Source: CAD feature listing. Evaluate the final solid. Frame: model axes, mm. Coordinates: 2 decimals unless noted, no trailing zeros. Order: outer loops, then holes, each group sorted by start corner. A loop starts at its lowest first (then second) coordinate and runs counter-clockwise, first axis right, second up. Notation, with made-up numbers: (12, 86.25) -> (45, 86.25) arc R19 ccw to (45, 104.25) -> close; hole circle Ø11 at (44.25, 40.25). An arc over 180 degrees is marked (long way). Write each question's results on one line, items separated by ' | '. Start each with the question number.
from build123d import *


with BuildPart() as part:
    # Sketch1 → Revolve1 (revolve)
    with BuildSketch(Plane.XY, mode=Mode.PRIVATE) as revolve1_sk:
        with BuildLine():
            Line((4, 25), (1, 25))
            Line((1, 25), (1, 0))
            Line((1, 0), (4, 0))
            ThreePointArc((4, 0), (6, 2), (4, 4))
            Line((4, 4), (3.5, 4))
            ThreePointArc((3.5, 4), (5, 7), (3.5, 10))
            Line((3.5, 10), (3.5, 15))
            ThreePointArc((3.5, 15), (5, 18), (3.5, 21))
            Line((3.5, 21), (4, 21))
            ThreePointArc((4, 21), (6, 23), (4, 25))
        make_face()
    revolve(revolve1_sk.sketch.rotate(Axis((0, 0, 0), (0, 1, 0)), 90), axis=Axis((0, 0, 0), (0, 1, 0)))


solid = part.part
(1) Draft query along X for faces 1 (the flat face through (1, 0, 1)), 2 (the cylindrical face through (1, 12, 0)), 3 (the cylindrical face through (3.105, 12.535, -1.615)). Return one class per face: released by +X, released by -X, zero draft, split by the parting line, or undercut.
(2) Line query: L1, parallel to X at y = 13, z = 0; L2, parallel to Y at x = 2.75, z = 3; L3, parallel to Z at x = -0.75, y = 18.75. Output: solid intervals per line, ascending.
(3) Section A-A on x = -3.75. Count the separate pieces of the cut face and the enclosed holes in it, then the cut area to 3 significant figures.
(4) First-contact query: P1, Ø5, axis at x = 0.5, y = 7.5, coming from the -Z side; P2, Ø4, axis at x = 1, y = 15, coming from the +Z side; P3, Ø1.5, axis at x = 2.5, y = 11.5, coming from the -Z side. Flat tips, straight axial feed; report the tip coordinate or a pass-through.
(5) Section B-B on y = 21.5. Return the cut outline in (x, z).
Results list:
1) face 1: zero draft | face 2: undercut | face 3: split by the parting line
2) L1: x = -3.5 to -1, 1 to 3.5 | L2: y = 0 to 4, 4.53 to 9.47, 15.53 to 20.47, 21 to 25 | L3: z = -4.87 to -0.66, 0.66 to 4.87
3) separate pieces: 4 | enclosed holes: 0 | area: 124 mm²
4) P1: stops at z = -5 | P2: stops at z = 4.82 | P3: stops at z = -3.03
5) outline: circle Ø10.65 at (0, 0); hole circle Ø2 at (0, 0)
